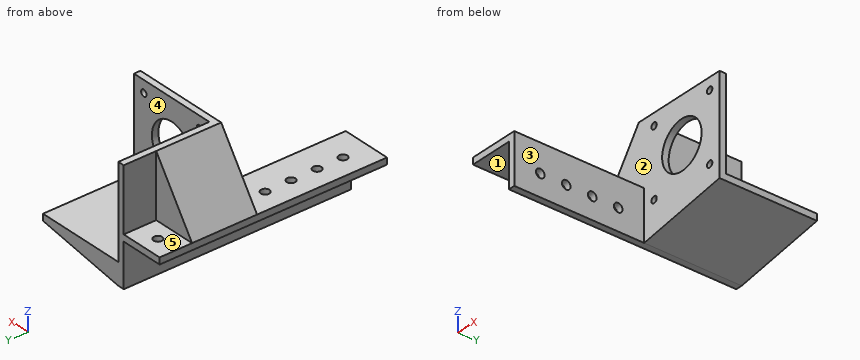
```python
from build123d import *

# Parameters (mm, degrees)
SKETCH1_W           = 42
SKETCH1_H           = 42
SKETCH1_R           = 11
SKETCH1_R_2         = 1.5
BOSS_EXTRUDE1_DEPTH = 3
BOSS_EXTRUDE2_DEPTH = 3
SKETCH4_W           = 42
SKETCH4_H           = 45
BOSS_EXTRUDE3_DEPTH = 3
BOSS_EXTRUDE4_DEPTH = 3
BOSS_EXTRUDE5_DEPTH = 30
SKETCH7_R           = 2
CUT_EXTRUDE1_DEPTH  = 24
BOSS_EXTRUDE6_DEPTH = 45
SKETCH9_R           = 2
CUT_EXTRUDE2_DEPTH  = 24


with BuildPart() as part:
    # Sketch1 → Boss-Extrude1 (new body)
    with BuildSketch(Plane(origin=(0, 0, 0), x_dir=(1, 0, 0), z_dir=(0, 1, 0))):
        Rectangle(SKETCH1_W, SKETCH1_H)
        Circle(SKETCH1_R, mode=Mode.SUBTRACT)
        with Locations((-15.5, -15.5)):
            Circle(SKETCH1_R_2, mode=Mode.SUBTRACT)
        with Locations((15.5, -15.5)):
            Circle(SKETCH1_R_2, mode=Mode.SUBTRACT)
        with Locations((-15.5, 15.5)):
            Circle(SKETCH1_R_2, mode=Mode.SUBTRACT)
        with Locations((15.5, 15.5)):
            Circle(SKETCH1_R_2, mode=Mode.SUBTRACT)
    extrude(amount=BOSS_EXTRUDE1_DEPTH)

    # Sketch2 → Boss-Extrude2 (add)
    with BuildSketch(Plane.ZY.offset(21)):
        Polygon((-11, 0), (-11, -60), (-31, -60), (-31, 45), (21, 45), (21, 0), align=None)
    extrude(amount=BOSS_EXTRUDE2_DEPTH)

    # Sketch4 → Boss-Extrude3 (add)
    with BuildSketch(Plane(origin=(0, 0, -21), x_dir=(-1, 0, 0), z_dir=(0, 0, -1))):
        with Locations((0, 22.5)):
            Rectangle(SKETCH4_W, SKETCH4_H)
    extrude(amount=BOSS_EXTRUDE3_DEPTH)

    # Sketch5 → Boss-Extrude4 (add)
    with BuildSketch(Plane.XY.offset(-11)):
        Polygon((-44, -60), (-21, -60), (-21, 0), (-24, 0), (-24, 45), (-44, 45), align=None)
    extrude(amount=BOSS_EXTRUDE4_DEPTH)

    # Sketch6 → Boss-Extrude5 (add)
    with BuildSketch(Plane.XZ):
        Polygon((-24, 21), (-44, -8), (-24, -8), align=None)
    extrude(amount=-BOSS_EXTRUDE5_DEPTH)

    # Sketch7 → Cut-Extrude1 (cut, through all)
    with BuildSketch(Plane.XY.offset(-8)):
        with Locations((-34, 37.5)):
            Circle(SKETCH7_R)
        with Locations((-34, -12)):
            Circle(SKETCH7_R)
        with Locations((-34, -24)):
            Circle(SKETCH7_R)
        with Locations((-34, -36)):
            Circle(SKETCH7_R)
        with Locations((-34, -48)):
            Circle(SKETCH7_R)
    extrude(amount=-CUT_EXTRUDE1_DEPTH, mode=Mode.SUBTRACT)

    # Sketch8 → Boss-Extrude6 (add)
    with BuildSketch(Plane.XZ):
        Polygon((21, -24), (-21, -31), (-21, -24), align=None)
    extrude(amount=-BOSS_EXTRUDE6_DEPTH)

    # Sketch9 → Cut-Extrude2 (cut, through all)
    with BuildSketch(Plane(origin=(-21, 0, 0), x_dir=(0, 0, -1), z_dir=(1, 0, 0))):
        with Locations((21, -12)):
            Circle(SKETCH9_R)
        with Locations((21, -24)):
            Circle(SKETCH9_R)
        with Locations((21, -36)):
            Circle(SKETCH9_R)
        with Locations((21, -48)):
            Circle(SKETCH9_R)
    extrude(amount=-CUT_EXTRUDE2_DEPTH, mode=Mode.SUBTRACT)


solid = part.part
```
Work out the finished part from the listing and answer in its coordinate system (mm). Face numbers are marked on the shaded views. A direction names the side the tool comes from. Give positions to 0.01 mm unless a question says otherwise; leave off trailing zeros. Order: outer loops, then holes, each group sorted by start corner. A loop starts at its lowest first (then second) coordinate and runs counter-clockwise, first axis right, second up.
1. Straight lines are drawn through the part: L1, parallel to Y at x = -34, z = -9; L2, parallel to Y at x = -22.1, z = -21; L3, parallel to Z at x = -15.5, y = 2.15. For each, find the intervals that lie inside material, in ascending order.
Result sheet:
L1: y = -60 to -50, -46 to -38, -34 to -26, -22 to -14, -10 to 35.5, 39.5 to 45
L2: y = -60 to -50, -46 to -38, -34 to -26, -22 to -14, -10 to 45
L3: z = -30.08 to -17, -14 to 14, 17 to 21
2. Section B-B, the plane y = 37.5 is taken. Determine the outline of the cut face in (x, z).
Result sheet:
outline: (-44, -11) - (-36, -11) - (-36, -8) - (-44, -8) - close; (-32, -11) - (-24, -11) - (-24, -31) - (-21, -31) - (21, -24) - (21, -21) - (-21, -21) - (-21, 21) - (-24, 21) - (-24, -8) - (-32, -8) - close
3. Each of these flat-tipped pins is pushed along its axis until it touches: P1, Ø11.5, axis at y = -36, z = -17.5, coming from the +X side; P2, Ø1, axis at x = -33.5, y = -5.5, coming from the +Z side; P3, Ø3.5, axis at x = -15.5, z = 15.5, coming from the -Y side. Where does it stop, or does it pass through?
Result sheet:
P1: stops at x = -21
P2: stops at z = -8
P3: stops at y = 0
4. Section C-C, the plane z = 5 is taken. Determine the outline of the cut face in (x, y).
Result sheet:
outline: (-35.03, 0) - (-9.8, 0) - (-9.8, 3) - (-21, 3) - (-21, 45) - (-24, 45) - (-24, 30) - (-35.03, 30) - close; (9.8, 0) - (21, 0) - (21, 3) - (9.8, 3) - close
5. Section D-D, the plane y = -48 is taken. Determine the outline of the cut face in (x, z), and give its area (3 significant figures).
Result sheet:
outline: (-44, -11) - (-36, -11) - (-36, -8) - (-44, -8) - close; (-32, -11) - (-24, -11) - (-24, -19) - (-21, -19) - (-21, -8) - (-32, -8) - close; (-24, -31) - (-21, -31) - (-21, -23) - (-24, -23) - close
area: 105 mm2
6. Section A-A, the plane x = 0 is taken. Determine the outline of the cut face in (y, z), and give its area (4 significant figures).
Result sheet:
outline: (0, -27.5) - (45, -27.5) - (45, -21) - (3, -21) - (3, -11) - (0, -11) - close; (0, 11) - (3, 11) - (3, 21) - (0, 21) - close
area: 352.5 mm2
7. For the marked faces 1, 2, 3, 4 and 5, determine the directions among +Z, -Z, +X, -X, +Y, -Y from which every point of the face is accessible in a straight line to the end or side of a thin tool.
Result sheet:
face 1: -Z, -X, +Y, -Y
face 2: +Z, +X, -Y
face 3: +Z, -Z, +X, -Y
face 4: +Z, +X, +Y
face 5: +Z, -X, +Y
